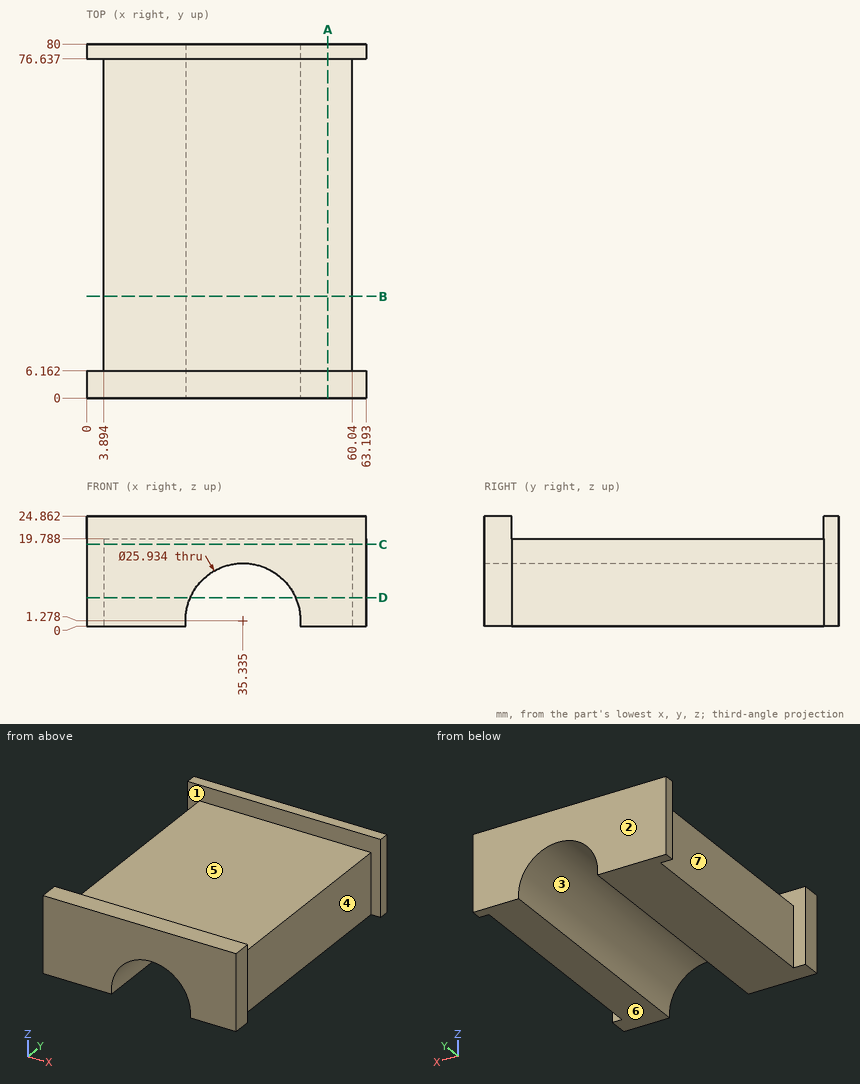
Can you work these out from the drawing? Everything is in mm from the part's minimum corner. A direction names the side the tool comes from. Round coordinates to 2 decimals unless told otherwise and drop trailing zeros. Loops run counter-clockwise (first coordinate to the right, second up) from the corner with the lowest first, then second, coordinate; pieces in that order, holes last. Notation, with made-up numbers: (40, 5) - (61, 5) arc R22 ccw to (61, 37) - close; hole circle Ø5 at (49.5, 25.5). An arc over 180 degrees is marked (long way). Answer in a Markdown table with one row per item. Add a question column.
Q1. We'd pull the mould along Y, two halves only. Please class the marked faces 1, 2, 3 and 4: pulls with the +Y half, pulls with the -Y half, needs draft (parallel to the pull), parting line crosses it, or undercut.
Q2. Which directions (+Z, -Z, +X, -X, +Y, -Y) give clear straight access to the entire face, cutting with the end or side of a thin tool? Please do the marked faces 5, 6 and 7.
Q3. I need wall thicknesses on L1, parallel to Y at x = 43, z = 20.25; L2, parallel to Z at x = 21, y = 46; L3, parallel to X at y = 16, z = 9.25 (1 decimal). Which ranges of each line are inside material? Lowest first, please.
Q4. For pin 1 Ø2 at (y, z) = (18.5, 18.5) entering from +X; pin 2 Ø1.5 at (x, y) = (38.5, 35) entering from -Z; pin 3 Ø5 at (x, y) = (16.5, 16) entering from +Z, each with a flat end and sliding along its axis, tell me the tip position at first contact or that it passes through.
Q5. I want a section at C-C on z = 18.5. List the corners of the cut face in (x, y) for me (1 decimal), and give its area (3 significant figures).
Q6. I want a section at A-A on x = 54.5. List the corners of the cut face in (y, z) for me, and give its area (3 significant figures).
Q7. I want a section at D-D on z = 6.5. List the corners of the cut face in (x, y) for me (1 decimal).
Q8. I want a section at B-B on y = 23. List the corners of the cut face in (x, z) for me (1 decimal).
A:
| question | item | result |
|---|---|---|
| 1 | face 1 | undercut |
| 1 | face 2 | pulls with the +Y half |
| 1 | face 3 | needs draft |
| 1 | face 4 | undercut |
| 2 | face 5 | +Z, +X, -X |
| 2 | face 6 | -Z, +X, -X, +Y, -Y |
| 2 | face 7 | +Z, -Z, -X |
| 3 | L1 | 0 to 6.16, 76.64 to 80 |
| 3 | L2 | 0 to 19.79 |
| 3 | L3 | 3.9 to 25.1, 45.6 to 60 |
| 4 | pin 1 | x = 60.04 |
| 4 | pin 2 | z = 13.64 |
| 4 | pin 3 | z = 19.79 |
| 5 | outline | (0, 0) - (63.2, 0) - (63.2, 6.2) - (60, 6.2) - (60, 76.6) - (63.2, 76.6) - (63.2, 80) - (0, 80) - (0, 76.6) - (3.9, 76.6) - (3.9, 6.2) - (0, 6.2) - close |
| 5 | area | 4,560 mm^2 |
| 6 | outline | (0, 0) - (80, 0) - (80, 24.86) - (76.64, 24.86) - (76.64, 19.79) - (6.16, 19.79) - (6.16, 24.86) - (0, 24.86) - close |
| 6 | area | 1,630 mm^2 |
| 7 | outline | (0, 0) - (23.5, 0) - (23.5, 80) - (0, 80) - (0, 76.6) - (3.9, 76.6) - (3.9, 6.2) - (0, 6.2) - close; (47.2, 0) - (63.2, 0) - (63.2, 6.2) - (60, 6.2) - (60, 76.6) - (63.2, 76.6) - (63.2, 80) - (47.2, 80) - close |
| 8 | outline | (3.9, 0) - (22.4, 0) arc R13 cw (long way) to (48.2, 0) - (60, 0) - (60, 19.8) - (3.9, 19.8) - close |
